The listing builds one solid part. Answer for the finished solid, in the listing's coordinates (mm). A direction names the side the tool comes from. Coordinates: 2 decimals unless noted, no trailing zeros. Write each loop counter-clockwise with the first axis right and the second up, starting at its lowest first coordinate (ties: lowest second). Pieces come first, ordered by that corner, then holes.
from build123d import *

# Parameters (mm, degrees)
F0_W     = 20
F0_H     = 40
F1_DEPTH = 500
F2_R     = 7.5
F2_R_2   = 5
F3_DEPTH = 25
F4_DEPTH = 25
F5_W     = 200
F5_H     = 10
F6_DEPTH = 40.001
F7_R     = 4


with BuildPart() as f1:
    # F0 (on Right) → F1 (new body, symmetric)
    with BuildSketch(Plane.YZ):
        Rectangle(F0_W, F0_H)
    extrude(amount=F1_DEPTH, both=True)

    # F2 (on face) → F3 (cut)
    with BuildSketch(Plane.XZ.offset(10)):
        with Locations((460, 0)):
            Circle(F2_R)
        with Locations((-475, 0)):
            Circle(F2_R_2)
        with Locations((-450, 0)):
            Circle(F2_R_2)
        with Locations((-425, 0)):
            Circle(F2_R_2)
        with Locations((-400, 0)):
            Circle(F2_R_2)
        with Locations((-375, 0)):
            Circle(F2_R_2)
    extrude(amount=-F3_DEPTH, mode=Mode.SUBTRACT)

    # F2 (on face) → F4 (cut)
    with BuildSketch(Plane.XZ.offset(10)):
        with Locations((460, 0)):
            Circle(F2_R)
        with Locations((-475, 0)):
            Circle(F2_R_2)
        with Locations((-450, 0)):
            Circle(F2_R_2)
        with Locations((-425, 0)):
            Circle(F2_R_2)
        with Locations((-400, 0)):
            Circle(F2_R_2)
        with Locations((-375, 0)):
            Circle(F2_R_2)
    extrude(amount=-F4_DEPTH, mode=Mode.SUBTRACT)

    # F5 (on face) → F6 (cut, through all)
    with BuildSketch(Plane.XY.offset(20)):
        with Locations((-400, 5)):
            Rectangle(F5_W, F5_H)
    extrude(amount=-F6_DEPTH, mode=Mode.SUBTRACT)

    # F7
    f7_edges = [f1.edges().sort_by_distance(p)[0] for p in [
        (-300, 0, 0),
    ]]
    fillet(f7_edges, radius=F7_R)


solid = f1.part
Q1. Which of the six approach directions +Z, -Z, +X, -X, +Y, -Y give full straight-line access (tool end or side, diameter ignored) to faces 1 (the face through (7, 0, -20)), 2 (the face through (-403, 0, 5))?
Answers below:
face 1: -Z, +X, -X, +Y, -Y
face 2: +Z, -Z, -X, +Y
Q2. The part is cut by section A-A, the plane x = -336. Write down the section's boundary in (y, z), then the cut area to 3 significant figures.
Answers below:
outline: (-10, -20) - (0, -20) - (0, 20) - (-10, 20) - close
area: 400 mm2
Q3. Find the intervals of material crossed by probe 1 along Z at (x, y) = (-375, -6); probe 2 along X at (y, z) = (5.25, 17); probe 3 along X at (y, z) = (-8.75, -6.5), in increasing order.
Answers below:
probe 1: z = -20 to -5, 5 to 20
probe 2: x = -300 to 500
probe 3: x = -500 to 456.26, 463.74 to 500
Q4. Given pin 1 (1 mm diameter, centred on y = 3.5, z = -9.5, fed in from -X); pin 2 (13 mm diameter, centred on x = -475, z = 0, fed in from +Y); pin 3 (1.8 mm diameter, centred on y = 6.5, z = 4, fed in from -X), each flat-ended and moving along its own axis, determine where each tip first touches the part or whether it passes through.
Answers below:
pin 1: stops at x = -300.13
pin 2: stops at y = 0
pin 3: stops at x = -300
